```python
from build123d import *

# Parameters (mm, degrees)
SKETCH1_W           = 20
SKETCH1_H           = 50
BOSS_EXTRUDE1_DEPTH = 20
CUT_EXTRUDE1_DEPTH  = 58.445626465
SKETCH3_R           = 5
CUT_EXTRUDE2_DEPTH  = 58.445626465
SKETCH4_R           = 5
CUT_EXTRUDE3_DEPTH  = 58.445626465
SKETCH5_R           = 0.5
CUT_EXTRUDE4_DEPTH  = 58.445626465


with BuildPart() as part:
    # Sketch1 → Boss-Extrude1 (new body)
    with BuildSketch(Plane.XY):
        with Locations((10, 25)):
            Rectangle(SKETCH1_W, SKETCH1_H)
    extrude(amount=-BOSS_EXTRUDE1_DEPTH)

    # Sketch2 → Cut-Extrude1 (cut, through all)
    with BuildSketch(Plane.XY):
        Polygon((20, 50), (20, 45), (15, 50), align=None)
    extrude(amount=-CUT_EXTRUDE1_DEPTH, mode=Mode.SUBTRACT)

    # Sketch3 → Cut-Extrude2 (cut, through all)
    with BuildSketch(Plane(origin=(20, 0, 0), x_dir=(0, 0, -1), z_dir=(1, 0, 0))):
        with Locations((10, 10)):
            Circle(SKETCH3_R)
    extrude(amount=-CUT_EXTRUDE2_DEPTH, mode=Mode.SUBTRACT)

    # Sketch4 → Cut-Extrude3 (cut, through all)
    with BuildSketch(Plane.XY):
        with Locations((10, 40)):
            Circle(SKETCH4_R)
    extrude(amount=-CUT_EXTRUDE3_DEPTH, mode=Mode.SUBTRACT)

    # Sketch5 → Cut-Extrude4 (cut, through all)
    with BuildSketch(Plane.XY):
        with Locations((20, 25)):
            Circle(SKETCH5_R)
    extrude(amount=-CUT_EXTRUDE4_DEPTH, mode=Mode.SUBTRACT)


solid = part.part
```
The model under review builds one solid part; all positions refer to its coordinate system, in mm. Coordinates: 2 decimals unless noted, no trailing zeros. Write each loop counter-clockwise with the first axis right and the second up, starting at its lowest first coordinate (ties: lowest second). Pieces come first, ordered by that corner, then holes.
1) Clearance check with a flat-ended pin moving along its axis: pin 1 Ø9 at (y, z) = (10, -10) entering from +X. State where the tip first meets the part, or that it passes through.
2) The part is to be moulded in two halves that separate along X. For faces 1 (the face through (13, 44, -10)), 2 (the face through (0, 25, -10)), 3 (the face through (10.14, 11.5, -14.77)), 4 (the face through (18, 47, -10)), say which applies: pulls with the +X half, pulls with the -X half, needs draft (parallel to the pull), parting line crosses it, or undercut.
3) To check wall thickness, follow probe 1 along Y at (x, z) = (10, -10.25); probe 2 along Y at (x, z) = (6.25, -10); probe 3 along Y at (x, z) = (15.25, -7.75). State the ranges of each line that lie inside material, in increasing order.
4) We need section C-C on y = 10. State the section outline as (x, z) points.
5) We need section B-B on x = 10. State the section outline as (y, z) points.
6) We need section A-A on z = -10. State the section outline as (x, y) points, then the cut area to 3 significant figures.
7) We need section D-D on z = -16.5. State the section outline as (x, y) points, then the cut area to 3 significant figures.
Answer list:
1. pin 1: passes through
2. face 1: undercut
2. face 2: pulls with the -X half
2. face 3: needs draft
2. face 4: pulls with the +X half
3. probe 1: y = 0 to 5.01, 14.99 to 35, 45 to 50
3. probe 2: y = 0 to 5, 15 to 36.69, 43.31 to 50
3. probe 3: y = 0 to 5.53, 14.47 to 49.75
4. outline: (0, -20) - (20, -20) - (20, -15) - (0, -15) - close; (0, -5) - (20, -5) - (20, 0) - (0, 0) - close
5. outline: (0, -20) - (35, -20) - (35, 0) - (0, 0) - close; (45, -20) - (50, -20) - (50, 0) - (45, 0) - close; hole circle Ø10 at (10, -10)
6. outline: (0, 0) - (20, 0) - (20, 5) - (0, 5) - close; (0, 15) - (20, 15) - (20, 24.5) arc R0.5 cw to (20, 25.5) - (20, 45) - (15, 50) - (0, 50) - close; hole circle Ø10 at (10, 40)
6. area: 709 mm2
7. outline: (0, 0) - (20, 0) - (20, 24.5) arc R0.5 cw to (20, 25.5) - (20, 45) - (15, 50) - (0, 50) - close; hole circle Ø10 at (10, 40)
7. area: 909 mm2
